Autodesk Inventor part; units mm, degrees
ref_plane "YZ Plane" through (0, 0, 0) normal (1, 0, 0) x (0, 1, 0)
ref_plane "XZ Plane" through (0, 0, 0) normal (0, 1, 0) x (-1, 0, 0)
ref_plane "XY Plane" through (0, 0, 0) normal (0, 0, 1) x (1, 0, 0)
sketch "Sketch1" plane through (0, 0, 0) normal (0, 1, 0) x (-1, 0, 0)
  line L0 (0, 0) -> (-100, 0)
  line L1 (-100, 0) -> (-100, -130)
  line L2 (-100, -130) -> (0, -130)
  line L3 (0, -130) -> (0, 0)
  dimension "Length" = 130
  dimension "Width" = 100
extrude "Baseplate" add sketch "Sketch1" along normal blind 3
sketch "TabsSketch" plane through (0, 3, 0) normal (0, 1, 0) x (1, 0, 0)
  line L0 (0, 130) -> (0, 0)
  line L1 (0, 20) -> (3, 20)
  line L2 (3, 20) -> (3, 40)
  line L3 (3, 40) -> (0, 40)
  line L4 (0, 40) -> (0, 20)
  line L5 (0, 90) -> (3, 90)
  line L6 (3, 90) -> (3, 110)
  line L7 (3, 110) -> (0, 110)
  line L8 (0, 110) -> (0, 90)
  line L9 (0, 0) -> (100, 0)
  line L10 (100, 130) -> (0, 130)
  line L11 (50, 0) -> (50, 130) construction
  line L12 (15, 0) -> (35, 0)
  line L13 (35, 0) -> (35, 3)
  line L14 (35, 3) -> (15, 3)
  line L15 (15, 3) -> (15, 0)
  line L16 (15, 130) -> (35, 130)
  line L17 (35, 130) -> (35, 127)
  line L18 (35, 127) -> (15, 127)
  line L19 (15, 127) -> (15, 130)
  line L20 (100, 130) -> (100, 0)
  line L21 (100, 20) -> (97, 20)
  line L22 (97, 20) -> (97, 40)
  line L23 (97, 40) -> (100, 40)
  line L24 (100, 40) -> (100, 20)
  line L25 (100, 90) -> (97, 90)
  line L26 (97, 90) -> (97, 110)
  line L27 (97, 110) -> (100, 110)
  line L28 (100, 110) -> (100, 90)
  line L29 (100, 0) -> (0, 0)
  line L30 (0, 130) -> (100, 130)
  line L31 (85, 0) -> (65, 0)
  line L32 (65, 0) -> (65, 3)
  line L33 (65, 3) -> (85, 3)
  line L34 (85, 3) -> (85, 0)
  line L35 (85, 130) -> (65, 130)
  line L36 (65, 130) -> (65, 127)
  line L37 (65, 127) -> (85, 127)
  line L38 (85, 127) -> (85, 130)
  point P0 (35, 0)
  point P1 (65, 0)
  point P2 (85, 0)
  point P3 (100, 110)
  point P4 (85, 130)
  point P5 (0, 110)
  point P6 (0, 40)
  dimension "d4" = 3
  dimension "LengthTabOffset" = 20
  dimension "d7" = 20
  dimension "d8" = 20
  dimension "BaseTabWidth" = 20
  dimension "d10" = 50
  dimension "d11" = 3
  dimension "d12" = 3
  dimension "d13" = 20
  dimension "d14" = 20
  dimension "WidthTabOffset" = 15
  dimension "d16" = 30
extrude "Extrusion2" cut sketch "TabsSketch" against normal through all contours L7 L6 L5 L0 | L10 L17 L18 L19 | L3 L2 L1 L0 | L10 L38 L37 L36 | L15 L14 L13 L9 | L20 L25 L26 L27 | L32 L33 L34 L9 | L20 L21 L22 L23
sketch "Sketch3" plane through (0, 3, 0) normal (0, 1, 0) x (1, 0, 0)
  circle A0 centre (10, 20) radius 1.6
  circle A1 centre (10, 109.5) radius 1.6
  circle A2 centre (91.5, 20) radius 1.6
  circle A3 centre (91.5, 109.5) radius 1.6
  line L0 (0, 20) -> (0, 0)
  line L1 (0, 90) -> (0, 40)
  line L2 (0, 0) -> (15, 0)
  line L3 (35, 0) -> (65, 0)
  circle A4 centre (23.5, 81.5) radius 1.6
  dimension "ScrewDiameter" = 3.2
  dimension "d20" = 3.2
  dimension "d21" = 3.2
  dimension "d22" = 3.2
  dimension "d23" = 89.5
  dimension "d24" = 81.5
  dimension "d25" = 89.5
  dimension "d26" = 81.5
  dimension "d27" = 10
  dimension "d28" = 10
  dimension "d29" = 20
  dimension "d30" = 20
  dimension "d31" = 61.5
  dimension "d32" = 68
  dimension "d33" = 3.2
extrude "PCB Mounting" cut sketch "Sketch3" against normal through all
equation "\"d4\" = Thickness"
equation "\"d7\" = LengthTabOffset"
equation "\"d8\" = BaseTabWidth"
equation "\"d11\" = Thickness"
equation "\"d12\" = Thickness"
equation "\"d13\" = BaseTabWidth"
equation "\"d14\" = BaseTabWidth"
equation "\"d20\" = ScrewDiameter"
equation "\"d21\" = ScrewDiameter"
equation "\"d22\" = d20"
equation "\"d25\" = d23"
equation "\"d26\" = d24"
equation "\"d28\" = d27"
equation "\"d30\" = d29"
equation "\"d33\" = ScrewDiameter"
properties part number "Base"
Can you work these out from the model? Positions are in its coordinate system, mm. A direction names the side the tool comes from. Coordinates: 2 decimals unless noted, no trailing zeros. Order: outer loops, then holes, each group sorted by start corner. A loop starts at its lowest first (then second) coordinate and runs counter-clockwise, first axis right, second up.
1. If we section it at C-C (y = 2.05): Give the number of separate pieces and of enclosed holes in the cut face, then the cut area to 3 significant figures.
2. Thinking about a two-plate mould opening in Z: for faces 1 (the face through (93, 1, -130)), 2 (the face through (100, 1, -65)), 3 (the face through (75, 2, -3)), 4 (the face through (98, 2, -40)), which applies, +Z half, -Z half, draft (parallel to the pull), parting line (faces both ways), or undercut?
3. If we section it at A-A (z = -81.5): Please give me the cut outline in (x, y).
4. For faces 5 (the face through (8, 1, -130)), 6 (the face through (3, 2, -30)), 7 (the face through (8.4, 1.52, -109.57)), 8 (the face through (35, 2, -1)), 9 (the face through (75, 2, -127)), which set-ups out of +Z, -Z, +X, -X, +Y, -Y let a thin tool reach every point of the face, with its end or its side?
5. I need wall thicknesses on line 1 (Z direction, x = 10, y = 1.55); line 2 (X direction, y = 2.35, z = -109.5); line 3 (Z direction, x = 34, y = 1.65). Which ranges of each line are inside material? Lowest first, please.
6. If we section it at B-B (x = 10): Please give me the cut outline in (y, z).
7. I'm going to push flat-ended pins straight in: pin 1 (0.9 mm diameter, centred on y = 2, z = -104.5, fed in from -X); pin 2 (1.5 mm diameter, centred on y = 1.5, z = -31.5, fed in from +X). Where does each tip first touch, or does it pass through?
8. If we section it at D-D (x = 69): Please give me the cut outline in (y, z), then the cut area to 3 significant figures.
Entries:
1. separate pieces: 1
1. enclosed holes: 5
1. area: 12,500 mm2
2. face 1: -Z half
2. face 2: draft
2. face 3: +Z half
2. face 4: undercut
3. outline: (0, 0) - (21.9, 0) - (21.9, 3) - (0, 3) - close; (25.1, 0) - (100, 0) - (100, 3) - (25.1, 3) - close
4. face 5: -Z, +X, -X, +Y, -Y
4. face 6: -X, +Y, -Y
4. face 7: +Y, -Y
4. face 8: +Z, +Y, -Y
4. face 9: -Z, +Y, -Y
5. line 1: z = -130 to -111.1, -107.9 to -21.6, -18.4 to 0
5. line 2: x = 3 to 8.4, 11.6 to 89.9, 93.1 to 97
5. line 3: z = -127 to -3
6. outline: (0, -130) - (3, -130) - (3, -111.1) - (0, -111.1) - close; (0, -107.9) - (3, -107.9) - (3, -21.6) - (0, -21.6) - close; (0, -18.4) - (3, -18.4) - (3, 0) - (0, 0) - close
7. pin 1: stops at x = 3
7. pin 2: stops at x = 97
8. outline: (0, -127) - (3, -127) - (3, -3) - (0, -3) - close
8. area: 372 mm2
